```python
from build123d import *

# Parameters (mm, degrees)
F0_W     = 100.0125
F0_H     = 80.16875
F1_DEPTH = 1.5875
F2_W     = 11.90625
F2_H     = 11.1125
F3_DEPTH = 3.175
F4_R     = 3.175
F5_DEPTH = 0.79375
F6_R     = 0.79375
F7_DEPTH = 25.4


with BuildPart() as f1:
    # F0 (on Top) → F1 (new body)
    with BuildSketch(Plane.XY):
        Rectangle(F0_W, F0_H)
    extrude(amount=F1_DEPTH)

    # F2 (on face) → F3 (join)
    with BuildSketch(Plane.XY.offset(1.5875)):
        with Locations((-17.065625, 32.940625)):
            Rectangle(F2_W, F2_H)
        with Locations((1.984375, 32.940625)):
            Rectangle(F2_W, F2_H)
        with Locations((21.034375, 32.940625)):
            Rectangle(F2_W, F2_H)
        Polygon((46.0375, 38.496875), (40.075645, 38.496875), (34.13125, 38.496875), (34.13125, 27.384375), (46.0375, 27.384375), align=None)
        with Locations((40.084375, 17.065625)):
            Rectangle(F2_W, F2_H)
        with Locations((40.084375, 1.190625)):
            Rectangle(F2_W, F2_H)
        with Locations((40.084375, -14.684375)):
            Rectangle(F2_W, F2_H)
        with Locations((40.084375, -30.559375)):
            Rectangle(F2_W, F2_H)
        with Locations((21.034375, -30.559375)):
            Rectangle(F2_W, F2_H)
        with Locations((1.984375, -30.559375)):
            Rectangle(F2_W, F2_H)
        Polygon((-23.01875, -25.003125), (-23.01875, -30.146314), (-23.01875, -36.115625), (-11.1125, -36.115625), (-11.1125, -25.003125), align=None)
        with Locations((-17.065625, -14.684375)):
            Rectangle(F2_W, F2_H)
        with Locations((-17.065625, 1.190625)):
            Rectangle(F2_W, F2_H)
        with Locations((-17.065625, 17.065625)):
            Rectangle(F2_W, F2_H)
        with Locations((1.984375, 17.065625)):
            Rectangle(F2_W, F2_H)
        with Locations((21.034375, 17.065625)):
            Rectangle(F2_W, F2_H)
        with Locations((21.034375, 1.190625)):
            Rectangle(F2_W, F2_H)
        with Locations((1.984375, 1.190625)):
            Rectangle(F2_W, F2_H)
        with Locations((1.984375, -14.684375)):
            Rectangle(F2_W, F2_H)
        with Locations((21.034375, -14.684375)):
            Rectangle(F2_W, F2_H)
    extrude(amount=F3_DEPTH)

    # F4 (on face) → F5 (join)
    with BuildSketch(Plane.XY.offset(4.7625)):
        with Locations((40.084375, -30.559375)):
            Circle(F4_R)
        with Locations((40.084375, -14.684375)):
            Circle(F4_R)
        with Locations((40.084375, 1.190625)):
            Circle(F4_R)
        with Locations((40.084375, 17.065625)):
            Circle(F4_R)
        with Locations((40.084375, 32.940625)):
            Circle(F4_R)
        with Locations((21.034375, 32.940625)):
            Circle(F4_R)
        with Locations((21.034375, 17.065625)):
            Circle(F4_R)
        with Locations((21.034375, 1.190625)):
            Circle(F4_R)
        with Locations((21.034375, -14.684375)):
            Circle(F4_R)
        with Locations((21.034375, -30.559375)):
            Circle(F4_R)
        with Locations((1.984375, -30.559375)):
            Circle(F4_R)
        with Locations((1.984375, -14.684375)):
            Circle(F4_R)
        with Locations((1.984375, 1.190625)):
            Circle(F4_R)
        with Locations((1.984375, 17.065625)):
            Circle(F4_R)
        with Locations((1.984375, 32.940625)):
            Circle(F4_R)
        with Locations((-17.065625, 32.940625)):
            Circle(F4_R)
        with Locations((-17.065625, 17.065625)):
            Circle(F4_R)
        with Locations((-17.065625, 1.190625)):
            Circle(F4_R)
        with Locations((-17.065625, -14.684375)):
            Circle(F4_R)
        with Locations((-17.065625, -30.559375)):
            Circle(F4_R)
    extrude(amount=F5_DEPTH)

    # F6 (on face) → F7 (cut)
    with BuildSketch(Plane.XY.offset(1.5875)):
        with Locations((-48.41875, 38.1)):
            Circle(F6_R)
        with Locations((48.815625, 38.1)):
            Circle(F6_R)
        with Locations((48.815625, -38.1)):
            Circle(F6_R)
    extrude(amount=-F7_DEPTH, mode=Mode.SUBTRACT)


solid = f1.part
```
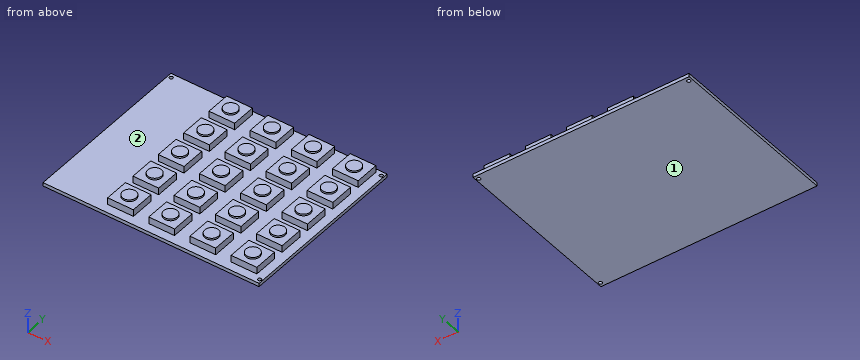
Geometry: final body of the model. Coordinates: model frame, mm. Face numbers are marked on the shaded views. Coordinates: 2 decimals unless noted, no trailing zeros. Write each loop counter-clockwise with the first axis right and the second up, starting at its lowest first coordinate (ties: lowest second). Pieces come first, ordered by that corner, then holes. Notation, with made-up numbers: M 77.25,78.5 L 124.25,78.5 A28 cw 124.25,101.5 Z; hole C 40.25,-16 d11. An arc over 180 degrees is marked long. Answer as CSV lines item,"result". Start each with the question number.
Q1. Mould query, pull axis X, two halves, no side actions, for the marked faces 1 and 2. Classes: released by +X, released by -X, zero draft, split by the parting line, or undercut.
Q2. Pin query (flat end, axial travel): P1, Ø4, axis at x = 32, y = -22, coming from the +Z side; P2, Ø1, axis at x = 23.5, z = 2.5, coming from the +Y side; P3, Ø1, axis at y = 17, z = 4, coming from the +X side. Return the tip coordinate at first contact, or that it passes through.
Q3. Line query: line 1 (X direction, y = 38.1, z = 1.25) (1 decimal); line 2 (Y direction, x = -13, z = 3.3); line 3 (X direction, y = 27.5, z = 4.4). Output: solid intervals per line, ascending. Write a range as from..to.
Q4. Cut plane B-B on x = 13.5. Return the cut outline in (y, z).
Q5. Cut plane A-A on z = 3.7. Count the separate pieces of the cut face and the enclosed holes in it, then the cut area to 3 significant figures.
Findings below:
1,face 1,"zero draft"
1,face 2,"undercut"
2,P1,"stops at z = 1.59"
2,P2,"stops at y = 38.5"
2,P3,"stops at x = 46.04"
3,line 1,"x = -50..-49.2, -47.6..48, 49.6..50"
3,line 2,"y = -36.12..-25, -20.24..-9.13, -4.37..6.75, 11.51..22.62, 27.38..38.5"
3,line 3,"x = -23.02..-11.11, -3.97..7.94, 15.08..26.99, 34.13..46.04"
4,outline,"M -40.08,0 L 40.08,0 L 40.08,1.59 L -40.08,1.59 Z"
5,separate pieces,"20"
5,enclosed holes,"0"
5,area,"2,650 mm2"
